```python
from build123d import *

# Parameters (mm, degrees)
EXTRUDE_1_DEPTH     = 4
CUT_EXTRUDE_1_DEPTH = 1
SKETCH_3_W          = 2
SKETCH_3_H          = 1
SKETCH_3_W_2        = 10.5
SKETCH_3_H_2        = 10.5
SKETCH_3_W_3        = 7.5
SKETCH_3_H_3        = 7.5
SKETCH_3_W_4        = 1
SKETCH_3_H_4        = 2
EXTRUDE_2_DEPTH     = 1
SKETCH_4_W          = 1.5
SKETCH_4_H          = 1.5
EXTRUDE_3_DEPTH     = 1


with BuildPart() as part:
    # Sketch 1 → Extrude 1 (new body)
    with BuildSketch(Plane(origin=(0, 0, 0), x_dir=(1, 0, 0), z_dir=(0, 1, 0))):
        Polygon((14.43375673, 0), (7.216878365, 12.5), (-7.216878365, 12.5), (-14.43375673, 0), (-7.216878365, -12.5), (7.216878365, -12.5), align=None)
    extrude(amount=EXTRUDE_1_DEPTH)

    # Sketch 2 → Cut-Extrude 1 (cut)
    with BuildSketch(Plane(origin=(0, 4, 0), x_dir=(1, 0, 0), z_dir=(0, 1, 0))):
        Polygon((5.484827557, -9.5), (10.969655115, 0), (5.484827557, 9.5), (-5.484827557, 9.5), (-10.969655115, 0), (-5.484827557, -9.5), align=None)
    extrude(amount=-CUT_EXTRUDE_1_DEPTH, mode=Mode.SUBTRACT)

    # Sketch 3 → Extrude 2 (add)
    # profile 1 of 21: a face of its own
    with BuildSketch(Plane(origin=(0, 3, 0), x_dir=(1, 0, 0), z_dir=(0, 1, 0))):
        with Locations((6.25, -4)):
            Rectangle(SKETCH_3_W, SKETCH_3_H)
    # profile 2 of 21: a face of its own
    with BuildSketch(Plane(origin=(0, 3, 0), x_dir=(1, 0, 0), z_dir=(0, 1, 0))):
        Rectangle(SKETCH_3_W_2, SKETCH_3_H_2)
        Rectangle(SKETCH_3_W_3, SKETCH_3_H_3, mode=Mode.SUBTRACT)
    # profile 3 of 21: a face of its own
    with BuildSketch(Plane(origin=(0, 3, 0), x_dir=(1, 0, 0), z_dir=(0, 1, 0))):
        with Locations((6.25, -2)):
            Rectangle(SKETCH_3_W, SKETCH_3_H)
    # profile 4 of 21: a face of its own
    with BuildSketch(Plane(origin=(0, 3, 0), x_dir=(1, 0, 0), z_dir=(0, 1, 0))):
        with Locations((6.25, 0)):
            Rectangle(SKETCH_3_W, SKETCH_3_H)
    # profile 5 of 21: a face of its own
    with BuildSketch(Plane(origin=(0, 3, 0), x_dir=(1, 0, 0), z_dir=(0, 1, 0))):
        with Locations((6.25, 2)):
            Rectangle(SKETCH_3_W, SKETCH_3_H)
    # profile 6 of 21: a face of its own
    with BuildSketch(Plane(origin=(0, 3, 0), x_dir=(1, 0, 0), z_dir=(0, 1, 0))):
        with Locations((6.25, 4)):
            Rectangle(SKETCH_3_W, SKETCH_3_H)
    # profile 7 of 21: a face of its own
    with BuildSketch(Plane(origin=(0, 3, 0), x_dir=(1, 0, 0), z_dir=(0, 1, 0))):
        with Locations((-6.25, 4)):
            Rectangle(SKETCH_3_W, SKETCH_3_H)
    # profile 8 of 21: a face of its own
    with BuildSketch(Plane(origin=(0, 3, 0), x_dir=(1, 0, 0), z_dir=(0, 1, 0))):
        with Locations((-6.25, 2)):
            Rectangle(SKETCH_3_W, SKETCH_3_H)
    # profile 9 of 21: a face of its own
    with BuildSketch(Plane(origin=(0, 3, 0), x_dir=(1, 0, 0), z_dir=(0, 1, 0))):
        with Locations((-6.25, 0)):
            Rectangle(SKETCH_3_W, SKETCH_3_H)
    # profile 10 of 21: a face of its own
    with BuildSketch(Plane(origin=(0, 3, 0), x_dir=(1, 0, 0), z_dir=(0, 1, 0))):
        with Locations((-6.25, -2)):
            Rectangle(SKETCH_3_W, SKETCH_3_H)
    # profile 11 of 21: a face of its own
    with BuildSketch(Plane(origin=(0, 3, 0), x_dir=(1, 0, 0), z_dir=(0, 1, 0))):
        with Locations((-6.25, -4)):
            Rectangle(SKETCH_3_W, SKETCH_3_H)
    # profile 12 of 21: a face of its own
    with BuildSketch(Plane(origin=(0, 3, 0), x_dir=(1, 0, 0), z_dir=(0, 1, 0))):
        with Locations((4, -6.25)):
            Rectangle(SKETCH_3_W_4, SKETCH_3_H_4)
    # profile 13 of 21: a face of its own
    with BuildSketch(Plane(origin=(0, 3, 0), x_dir=(1, 0, 0), z_dir=(0, 1, 0))):
        with Locations((2, -6.25)):
            Rectangle(SKETCH_3_W_4, SKETCH_3_H_4)
    # profile 14 of 21: a face of its own
    with BuildSketch(Plane(origin=(0, 3, 0), x_dir=(1, 0, 0), z_dir=(0, 1, 0))):
        with Locations((0, -6.25)):
            Rectangle(SKETCH_3_W_4, SKETCH_3_H_4)
    # profile 15 of 21: a face of its own
    with BuildSketch(Plane(origin=(0, 3, 0), x_dir=(1, 0, 0), z_dir=(0, 1, 0))):
        with Locations((-2, -6.25)):
            Rectangle(SKETCH_3_W_4, SKETCH_3_H_4)
    # profile 16 of 21: a face of its own
    with BuildSketch(Plane(origin=(0, 3, 0), x_dir=(1, 0, 0), z_dir=(0, 1, 0))):
        with Locations((-4, -6.25)):
            Rectangle(SKETCH_3_W_4, SKETCH_3_H_4)
    # profile 17 of 21: a face of its own
    with BuildSketch(Plane(origin=(0, 3, 0), x_dir=(1, 0, 0), z_dir=(0, 1, 0))):
        with Locations((-4, 6.25)):
            Rectangle(SKETCH_3_W_4, SKETCH_3_H_4)
    # profile 18 of 21: a face of its own
    with BuildSketch(Plane(origin=(0, 3, 0), x_dir=(1, 0, 0), z_dir=(0, 1, 0))):
        with Locations((-2, 6.25)):
            Rectangle(SKETCH_3_W_4, SKETCH_3_H_4)
    # profile 19 of 21: a face of its own
    with BuildSketch(Plane(origin=(0, 3, 0), x_dir=(1, 0, 0), z_dir=(0, 1, 0))):
        with Locations((0, 6.25)):
            Rectangle(SKETCH_3_W_4, SKETCH_3_H_4)
    # profile 20 of 21: a face of its own
    with BuildSketch(Plane(origin=(0, 3, 0), x_dir=(1, 0, 0), z_dir=(0, 1, 0))):
        with Locations((2, 6.25)):
            Rectangle(SKETCH_3_W_4, SKETCH_3_H_4)
    # profile 21 of 21: a face of its own
    with BuildSketch(Plane(origin=(0, 3, 0), x_dir=(1, 0, 0), z_dir=(0, 1, 0))):
        with Locations((4, 6.25)):
            Rectangle(SKETCH_3_W_4, SKETCH_3_H_4)
    extrude(amount=EXTRUDE_2_DEPTH)

    # Sketch 4 → Extrude 3 (add)
    with BuildSketch(Plane(origin=(0, 3, 0), x_dir=(1, 0, 0), z_dir=(0, 1, 0))):
        with Locations((-2.335786438, -2.335786438)):
            Rectangle(SKETCH_4_W, SKETCH_4_H)
    extrude(amount=EXTRUDE_3_DEPTH)


solid = part.part
```
Can you work these out from the model? Positions are in its coordinate system, mm. Give positions to 0.01 mm unless a question says otherwise; leave off trailing zeros. Loops run counter-clockwise (first coordinate to the right, second up) from the corner with the lowest first, then second, coordinate; pieces in that order, holes last. Notation, with made-up numbers: M 80,61.25 L 99,61.25 A22 ccw 99,73.25 Z; hole C -21,33.25 d1. An arc over 180 degrees is marked long. One line per question, with ' | ' between items. Start each with the question number.
Q1. If we section it at A-A (y = 3.4): State how many separate pieces and enclosed holes the cut face has, plus the area to 3 significant figures.
Q2. If we section it at B-B (x = -1): Please give me the cut outline in (y, z), plus the area to 3 significant figures.
Q3. If we section it at C-C (z = 8): Please give me the cut outline in (x, y).
Q4. For pin 1 Ø6 at (x, z) = (7.5, -5.5) entering from +Y; pin 2 Ø0.5 at (y, z) = (3.5, 6) entering from -X; pin 3 Ø1 at (y, z) = (3, 5.5) entering from +X; pin 4 Ø2 at (y, z) = (1, -7) entering from -X, each with a flat end and sliding along its axis, tell me the tip position at first contact or that it passes through.
Q5. If I drill on line 1 (Y direction, x = -5.75, z = -7); line 2 (Z direction, x = -9.75, y = 3.35); line 3 (X direction, y = 3.4, z = 1.75), over which ranges is the centre line in solid material (lowest first)? Write a range as from..to.
Q6. If we section it at D-D (y = 1.25): Please give me the cut outline in (x, z), plus the area to 3 significant figures.
Computed:
1) separate pieces: 3 | enclosed holes: 2 | area: 325 mm²
2) outline: M 0,-12.5 L 4,-12.5 L 4,-9.5 L 3,-9.5 L 3,-5.25 L 4,-5.25 L 4,-3.75 L 3,-3.75 L 3,3.75 L 4,3.75 L 4,5.25 L 3,5.25 L 3,9.5 L 4,9.5 L 4,12.5 L 0,12.5 Z | area: 84.0 mm²
3) outline: M -9.81,0 L 9.81,0 L 9.81,4 L 6.35,4 L 6.35,3 L -6.35,3 L -6.35,4 L -9.81,4 Z
4) pin 1: stops at y = 4 | pin 2: stops at x = -11.11 | pin 3: stops at x = 11.55 | pin 4: stops at x = -10.97
5) line 1: y = 0..3 | line 2: z = -8.11..-2.11, 2.11..8.11 | line 3: x = -13.42..-9.96, -7.25..-3.75, -3.09..-1.59, 3.75..7.25, 9.96..13.42
6) outline: M -14.43,0 L -7.22,-12.5 L 7.22,-12.5 L 14.43,0 L 7.22,12.5 L -7.22,12.5 Z | area: 541 mm²
